Build history of the part. All positions in model axes, mm. A direction names the side the tool comes from. Round coordinates to 2 decimals unless told otherwise and drop trailing zeros. Write each loop counter-clockwise with the first axis right and the second up, starting at its lowest first coordinate (ties: lowest second). Pieces come first, ordered by that corner, then holes. Notation, with made-up numbers: (-18, 9) -> (34, 9) arc R18 ccw to (34, 34) -> close; hole circle Ø7 at (29.25, 48.5). An arc over 180 degrees is marked (long way). Return JSON: item names as keys, results as strings.
from build123d import *

# Parameters (mm, degrees)
SKETCH1_R      = 1.75
SKETCH1_R_2    = 4.25
SKETCH1_R_3    = 10
SKETCH1_W      = 8.5
SKETCH1_H      = 20.5
SKETCH1_H_2    = 15.5
SKETCH1_H_3    = 8.5
EXTRUDE1_DEPTH = 8


with BuildPart() as part:
    # Sketch1 → Extrude1 (new body)
    with BuildSketch(Plane.XY):
        with BuildLine():
            Line((234.88475828, 56.014964012), (234.88475828, 44.014964012))
            Line((234.88475828, 44.014964012), (254.88475828, 44.014964012))
            Line((254.88475828, 44.014964012), (254.88475828, 59.014964012))
            Line((254.88475828, 59.014964012), (268.88475828, 59.014964012))
            ThreePointArc((268.88475828, 59.014964012), (273.127398968, 57.257604699), (274.88475828, 53.014964012))
            Line((274.88475828, 53.014964012), (274.88475828, 11.014964012))
            ThreePointArc((274.88475828, 11.014964012), (273.127398968, 6.772323325), (268.88475828, 5.014964012))
            Line((268.88475828, 5.014964012), (234.88475828, 5.014964012))
            Line((234.88475828, 5.014964012), (231.88475828, 8.014964012))
            Line((231.88475828, 8.014964012), (47.88475828, 8.014964012))
            Line((47.88475828, 8.014964012), (44.88475828, 5.014964012))
            Line((44.88475828, 5.014964012), (10.88475828, 5.014964012))
            ThreePointArc((10.88475828, 5.014964012), (6.642117593, 6.772323325), (4.88475828, 11.014964012))
            Line((4.88475828, 11.014964012), (4.88475828, 53.014964012))
            ThreePointArc((4.88475828, 53.014964012), (6.642117593, 57.257604699), (10.88475828, 59.014964012))
            Line((10.88475828, 59.014964012), (24.88475828, 59.014964012))
            Line((24.88475828, 59.014964012), (24.88475828, 44.014964012))
            Line((24.88475828, 44.014964012), (44.88475828, 44.014964012))
            Line((44.88475828, 44.014964012), (44.88475828, 56.014964012))
            ThreePointArc((44.88475828, 56.014964012), (45.763437937, 58.136284356), (47.88475828, 59.014964012))
            Line((47.88475828, 59.014964012), (231.88475828, 59.014964012))
            ThreePointArc((231.88475828, 59.014964012), (234.006078624, 58.136284356), (234.88475828, 56.014964012))
        make_face()
        with Locations((260.38475828, 47.014964012)):
            Circle(SKETCH1_R, mode=Mode.SUBTRACT)
        with Locations((260.38475828, 17.014964012)):
            Circle(SKETCH1_R, mode=Mode.SUBTRACT)
        with Locations((19.38475828, 47.014964012)):
            Circle(SKETCH1_R, mode=Mode.SUBTRACT)
        with Locations((19.38475828, 17.014964012)):
            Circle(SKETCH1_R, mode=Mode.SUBTRACT)
        with Locations((224.38475828, 50.514964012)):
            Circle(SKETCH1_R_2, mode=Mode.SUBTRACT)
        with Locations((224.38475828, 24.514964012)):
            Circle(SKETCH1_R_2, mode=Mode.SUBTRACT)
        with Locations((55.38475828, 50.514964012)):
            Circle(SKETCH1_R_2, mode=Mode.SUBTRACT)
        with Locations((55.38475828, 24.514964012)):
            Circle(SKETCH1_R_2, mode=Mode.SUBTRACT)
        with Locations((191.88475828, 15.514964012)):
            Circle(SKETCH1_R, mode=Mode.SUBTRACT)
        with Locations((191.88475828, 45.514964012)):
            Circle(SKETCH1_R, mode=Mode.SUBTRACT)
        with Locations((151.88475828, 15.514964012)):
            Circle(SKETCH1_R, mode=Mode.SUBTRACT)
        with Locations((151.88475828, 45.514964012)):
            Circle(SKETCH1_R, mode=Mode.SUBTRACT)
        with Locations((81.38475828, 38.514964012)):
            Circle(SKETCH1_R, mode=Mode.SUBTRACT)
        with Locations((70.38475828, 50.514964012)):
            Circle(SKETCH1_R, mode=Mode.SUBTRACT)
        with Locations((134.88475828, 41.514964012)):
            Circle(SKETCH1_R_3, mode=Mode.SUBTRACT)
        with Locations(Location((209.38475828, 50.514964012, 0), (0, 0, 180))):
            Circle(SKETCH1_R, mode=Mode.SUBTRACT)
        with Locations((260.38475828, 32.014964012)):
            Rectangle(SKETCH1_W, SKETCH1_H, mode=Mode.SUBTRACT)
        with Locations((19.38475828, 32.014964012)):
            Rectangle(SKETCH1_W, SKETCH1_H, mode=Mode.SUBTRACT)
        with Locations((191.88475828, 30.514964012)):
            Rectangle(SKETCH1_W, SKETCH1_H_2, mode=Mode.SUBTRACT)
        with Locations((151.88475828, 30.514964012)):
            Rectangle(SKETCH1_W, SKETCH1_H_2, mode=Mode.SUBTRACT)
        with Locations((67.38475828, 38.514964012)):
            Rectangle(SKETCH1_W, SKETCH1_H_3, mode=Mode.SUBTRACT)
    extrude(amount=EXTRUDE1_DEPTH)


solid = part.part
Q1. 3-axis set-ups, long thin cutter, end or side, ignore diameter. For faces 1 (the flat face through (245, 44.015, 4)), 2 (the flat face through (152, 38.265, 4)), 3 (the cylindrical face through (6.689, 6.726, 3.944)): which of +Z, -Z, +X, -X, +Y, -Y reach the whole face in a straight line?
Verdict:
{"face 1": "+Z, -Z, +Y", "face 2": "+Z, -Z", "face 3": "+Z, -Z, -X, -Y"}
Q2. Saw through at C-C on z = 5. Count the separate pieces of the cut face and the enclosed holes in it, then the cut area to 3 significant figures.
Verdict:
{"separate pieces": "1", "enclosed holes": "21", "area": "12,100 mm²"}
Q3. Saw through at B-B on x = 182. List the corners of the cut face in (y, z), then the cut area to 3 significant figures.
Verdict:
{"outline": "(8.01, 0) -> (59.01, 0) -> (59.01, 8) -> (8.01, 8) -> close", "area": "408 mm²"}
Q4. Wall check: L1, parallel to X at y = 29, z = 2.5; L2, parallel to Y at x = 149, z = 7.25; L3, parallel to X at y = 17.5, z = 7.75. Give the ranges that are in metal, low to high.
Verdict:
{"L1": "x = 4.88 to 15.13, 23.63 to 147.63, 156.13 to 187.63, 196.13 to 256.13, 264.63 to 274.88", "L2": "y = 8.01 to 22.76, 38.26 to 59.01", "L3": "x = 4.88 to 17.7, 21.07 to 258.7, 262.07 to 274.88"}
Q5. Saw through at A-A on x = 142.5. List the corners of the cut face in (y, z).
Verdict:
{"outline": "(8.01, 0) -> (35.03, 0) -> (35.03, 8) -> (8.01, 8) -> close; (48, 0) -> (59.01, 0) -> (59.01, 8) -> (48, 8) -> close"}
Q6. Saw through at D-D on x = 38.5. List the corners of the cut face in (y, z), then the cut area to 3 significant figures.
Verdict:
{"outline": "(5.01, 0) -> (44.01, 0) -> (44.01, 8) -> (5.01, 8) -> close", "area": "312 mm²"}
Q7. Pin check, flat tip, straight feed: pin 1 Ø2.5 at (x, z) = (154, 5) entering from -Y. Stop position of the tip, or through.
Verdict:
{"pin 1": "stops at y = 8.01"}
Q8. Two-plate mould, pull along X, no slides. Class faces 4 (the cylindrical face through (273.174, 6.819, 3.944)), 5 (the flat face through (35, 44.015, 4)), 6 (the flat face through (142, 32, 8)): +X half, -X half, draft (parallel to the pull), parting line (faces both ways), or undercut.
Verdict:
{"face 4": "+X half", "face 5": "undercut", "face 6": "draft"}
